```python
from build123d import *

# Parameters (mm, degrees)
F0_W     = 15.2882066071
F0_H     = 15.2716501616
F0_H_2   = 12.5766545534
F0_W_2   = 86.0167954564
F0_H_3   = 6.9620762952
F1_DEPTH = 1.5
F0_W_3   = 0.6571944356
F0_W_4   = 0.4326078594
F2_DEPTH = 15
F3_SIZE  = 2


with BuildPart() as f1:
    # F0 (on Top) → F1 (new body)
    with BuildSketch(Plane.XY):
        Polygon((52, 14.529729262), (52, 24.5), (-52, 24.5), (-52, 14.529729262), (-36.7117933929, 14.529729262), (-36.7117933929, 1.9530747086), (-52, 1.9530747086), (-52, -2.5385871995), (-36.7117933929, -2.5385871995), (-36.7117933929, -17.8102373611), (-52, -17.8102373611), (-52, -24.5), (52, -24.5), (52, -14.529729262), (-34.0167954564, -14.529729262), (-34.0167954564, -7.5676529668), (52, -7.5676529668), (52, 7.5676529668), (-34.0167954564, 7.5676529668), (-34.0167954564, 14.529729262), align=None)
        with Locations((-44.3558966964, -10.1744122803)):
            Rectangle(F0_W, F0_H)
        with Locations((-44.3558966964, 8.2414019853)):
            Rectangle(F0_W, F0_H_2)
        with Locations((8.9916022718, 11.0486911144)):
            Rectangle(F0_W_2, F0_H_3)
        with Locations((8.9916022718, -11.0486911144)):
            Rectangle(F0_W_2, F0_H_3)
    extrude(amount=F1_DEPTH)

    # F0 (on Top) → F2 (join)
    with BuildSketch(Plane.XY):
        with Locations((-44.3558966964, 8.2414019853)):
            Rectangle(F0_W, F0_H_2)
        with Locations((-44.3558966964, -10.1744122803)):
            Rectangle(F0_W, F0_H)
        with Locations((-52.3285972178, -10.1744122803)):
            Rectangle(F0_W_3, F0_H)
        with Locations((-52.2163039297, 8.2414019853)):
            Rectangle(F0_W_4, F0_H_2)
        with Locations((8.9916022718, 11.0486911144)):
            Rectangle(F0_W_2, F0_H_3)
        with Locations((8.9916022718, -11.0486911144)):
            Rectangle(F0_W_2, F0_H_3)
    extrude(amount=F2_DEPTH)

    # F3
    f3_edges = [f1.edges().sort_by_distance(p)[0] for p in [
        (8.991602, -7.567653, 15),
        (8.991602, 7.567653, 15),
    ]]
    chamfer(f3_edges, length=F3_SIZE)


solid = f1.part
```
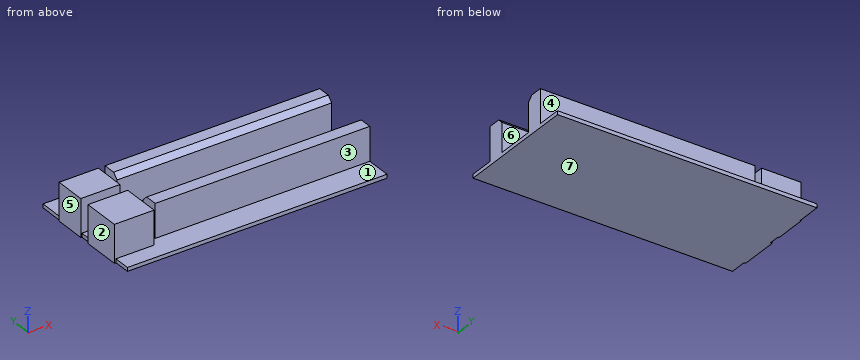
Read the model definition and answer for the solid it produces. Units are mm, in the model's axes. Face numbers are marked on the shaded views. A direction names the side the tool comes from. Coordinates: 2 decimals unless noted, no trailing zeros. Order: outer loops, then holes, each group sorted by start corner. A loop starts at its lowest first (then second) coordinate and runs counter-clockwise, first axis right, second up. Notation, with made-up numbers: (-14.5, -36.75) - (34.5, -36.75) arc R23 ccw to (34.5, -2.75) - close; hole circle Ø11 at (-15.75, 37). An arc over 180 degrees is marked (long way). Answer as a JSON object with one key per item and string values. Group by question number.
Item 1: Section B-B (x = 31.5) is taken. Give the vertices of the cut face in (y, z), plus the area to 3 significant figures.
Item 2: Section A-A (z = 4.5) is taken. Give the vertices of the cut face in (x, y), plus the area to 3 significant figures.
Item 3: Consider probe 1 along Y at (x, z) = (-37, 2.5); probe 2 along Y at (x, z) = (-20.5, 11); probe 3 along X at (y, z) = (-10, 5.25). Determine where each line is inside the solid, lowest interval first. Write a range as from..to.
Item 4: Flat-ended cylindrical pins translate along their axes: P1, Ø1.2, axis at y = -22.5, z = 1, coming from the -X side; P2, Ø4, axis at x = 34.5, z = 7, coming from the -Y side; P3, Ø4, axis at y = 3.5, z = 1.5, coming from the -X side; P4, Ø1, axis at y = -1.5, z = 6, coming from the +X side. Find the tip coordinate at first contact, or state that the pin passes through.
Item 5: Section C-C (y = 17) is taken. Give the vertices of the cut face in (x, z), plus the area to 3 significant figures.
Item 6: The mould has two halves that part along Y. Classify the marked faces 1, 2, 3 and 4: +Y half, -Y half, draft (parallel to the pull), parting line (faces both ways), or undercut.
Item 7: Section D-D (x = -38) is taken. Give the vertices of the cut face in (y, z).
Item 8: A tool of negligible diameter and unlimited length cuts with its end or side. For the marked faces 5, 6 and 7, from which of +Z, -Z, +X, -X, +Y, -Y can it reach the whole face along a straight path? Write none if from no direction.
Results are:
{
 "1": {"outline": "(-24.5, 0) - (24.5, 0) - (24.5, 1.5) - (14.53, 1.5) - (14.53, 15) - (9.57, 15) - (7.57, 13) - (7.57, 1.5) - (-7.57, 1.5) - (-7.57, 13) - (-9.57, 15) - (-14.53, 15) - (-14.53, 1.5) - (-24.5, 1.5) - close", "area": "257 mm^2"},
 "2": {"outline": "(-52.66, -17.81) - (-36.71, -17.81) - (-36.71, -2.54) - (-52.66, -2.54) - close; (-52.43, 1.95) - (-36.71, 1.95) - (-36.71, 14.53) - (-52.43, 14.53) - close; (-34.02, -14.53) - (52, -14.53) - (52, -7.57) - (-34.02, -7.57) - close; (-34.02, 7.57) - (52, 7.57) - (52, 14.53) - (-34.02, 14.53) - close", "area": "1,640 mm^2"},
 "3": {"probe 1": "y = -17.81..-2.54, 1.95..14.53", "probe 2": "y = -14.53..-7.57, 7.57..14.53", "probe 3": "x = -52.66..-36.71, -34.02..52"},
 "4": {"P1": "stops at x = -52", "P2": "stops at y = -14.53", "P3": "stops at x = -52.43", "P4": "passes through"},
 "5": {"outline": "(-52, 0) - (52, 0) - (52, 1.5) - (-52, 1.5) - close", "area": "156 mm^2"},
 "6": {"face 1": "undercut", "face 2": "draft", "face 3": "-Y half", "face 4": "+Y half"},
 "7": {"outline": "(-24.5, 0) - (24.5, 0) - (24.5, 1.5) - (14.53, 1.5) - (14.53, 15) - (1.95, 15) - (1.95, 1.5) - (-2.54, 1.5) - (-2.54, 15) - (-17.81, 15) - (-17.81, 1.5) - (-24.5, 1.5) - close"},
 "8": {"face 5": "+Z, -Z, -X, +Y", "face 6": "+Z, +X", "face 7": "-Z, +X, -X, +Y, -Y"}
}
